```python
from build123d import *

# Parameters (mm, degrees)
EXTRUDE_1_DEPTH          = 66
CUT_EXTRUDE_1_DEPTH      = 66
CUT_EXTRUDE_1_DEPTH_BACK = 66
SKETCH_2_R               = 1.5
SKETCH_4_R               = 3.5
CUT_EXTRUDE_2_DEPTH      = 5
CUT_EXTRUDE_3_DEPTH      = 66
REVOLVE_1_ANGLE          = 110
SKETCH_7_W               = 6.196152423
SKETCH_7_H               = 4
CUT_EXTRUDE_4_DEPTH      = 66


with BuildPart() as part:
    # 草图1 → 凸台-拉伸1 (new body)
    with BuildSketch(Plane(origin=(0, 0, 0), x_dir=(0, 0, -1), z_dir=(1, 0, 0))):
        Polygon((5, 0), (-5, 0), (-25, 34.641016151), (-21.535898385, 36.641016151), (-7.25388745, 11.903847577), (-2, 11.903847577), (-2, 2.803847577), (2, 2.803847577), (2, 11.903847577), (7.25388745, 11.903847577), (21.535898385, 36.641016151), (25, 34.641016151), align=None)
    extrude(amount=EXTRUDE_1_DEPTH)

    # 草图2 → 切除-拉伸1 (cut, two sides: drawn at the far end of the back side and taken through both)
    with BuildSketch(Plane.XY.offset(-CUT_EXTRUDE_1_DEPTH_BACK)):
        with Locations(Location((5, 8.23, 0), (0, 0, 180))):
            Circle(SKETCH_2_R)
        with Locations(Location((50, 8.23, 0), (0, 0, 180))):
            Circle(SKETCH_2_R)
        Polygon((0, 9), (0, 36.641016151), (75.943067727, 36.641016151), (66, 33.022035462), (66, 0), (55.386922379, 29.159191114), align=None)
    extrude(amount=CUT_EXTRUDE_1_DEPTH + CUT_EXTRUDE_1_DEPTH_BACK, mode=Mode.SUBTRACT)

    # 草图4 → 切除-拉伸2 (cut)
    with BuildSketch(Plane(origin=(0, 0, 12), x_dir=(-1, 0, 0), z_dir=(0, 0, -1))):
        with Locations((-5, 8.23)):
            Circle(SKETCH_4_R)
        with Locations(Location((-50, 8.23, 0), (0, 0, 90))):
            Circle(SKETCH_4_R)
    cut_extrude_2 = extrude(amount=CUT_EXTRUDE_2_DEPTH, mode=Mode.SUBTRACT)

    # 镜向1: 切除-拉伸2 across plane
    add(cut_extrude_2.mirror(Plane.XY), mode=Mode.SUBTRACT)

    # 草图5 → 切除-拉伸3 (cut)
    with BuildSketch(Plane(origin=(0, -2.165063509, 3.75), x_dir=(1, 0, 0), z_dir=(0, -0.5000000000000011, 0.8660254037844382))):
        Polygon((32.339646553, 26.483902367), (34.276892815, 21.874447202), (51.364505918, 22.320217945), (58.994441321, 24.725230573), (55.386922379, 36.170133678), align=None)
    cut_extrude_3 = extrude(amount=-CUT_EXTRUDE_3_DEPTH, mode=Mode.SUBTRACT)

    # 镜向2: 切除-拉伸3 across plane
    add(cut_extrude_3.mirror(Plane.XY), mode=Mode.SUBTRACT)

    # 草图6 → 旋转1 (revolve)
    with BuildSketch(Plane.ZY):
        Polygon((-10.196152423, 9), (-2, 9), (-2, 2.803847577), (2, 2.803847577), (2, 9), (10.196152423, 9), (5, 0), (-5, 0), align=None)
    revolve(axis=Axis((0, 9, -10.196152423), (0, 0, -1)), revolution_arc=REVOLVE_1_ANGLE)

    # 草图7 → 切除-拉伸4 (cut)
    with BuildSketch(Plane(origin=(2.892544244, 7.947199994, 0), x_dir=(0.939692620785907, -0.34202014332567265, 0), z_dir=(0.34202014332567265, 0.939692620785907, 0))):
        with Locations((-6.176257502, 0)):
            Rectangle(SKETCH_7_W, SKETCH_7_H)
    extrude(amount=-CUT_EXTRUDE_4_DEPTH, mode=Mode.SUBTRACT)


solid = part.part
```
Design review of the part built by this model. Coordinates are the model's own, in mm. A direction names the side the tool comes from. Coordinates: 2 decimals unless noted, no trailing zeros. Order: outer loops, then holes, each group sorted by start corner. A loop starts at its lowest first (then second) coordinate and runs counter-clockwise, first axis right, second up.
1) Clearance check with flat-ended pins moving along their axes: pin 1 (11 mm diameter, centred on x = 50, y = 8.23, fed in from +Z); pin 2 (10 mm diameter, centred on y = 13, z = -10.5, fed in from -X); pin 3 (4 mm diameter, centred on x = 22, z = 4.5, fed in from +Y); pin 4 (6 mm diameter, centred on y = 18, z = 4.5, fed in from -X). State where each tip first meets the part, or that it passes through.
2) Wall thickness on line 1 along X through (y, z) = (8.23, 9.25); line 2 along X through (y, z) = (7.5, 3); line 3 along Z through (x, y) = (58, 10.75): over which ranges is each line inside the solid? List them lowest first.
3) Mouldability with a two-part tool opening along X and no side actions: class faces 6 (the conical face through (-3.7, 6.33, 7.56)), 7 (the flat face through (28, 7, -2)), 8 (the flat face through (55.126, 19.178, 13.795)) as +X half, -X half, draft (parallel to the pull), parting line (faces both ways), or undercut.
4) Take a section at D-D, the plane x = 29. Give the boundary of the cut face in (y, z).
5) Take a section at B-B, the plane z = 0. Give the boundary of the cut face in (x, y) (3 decimals).
6) Take a section at A-A, the plane y = 13.75. Give the boundary of the cut face in (x, z), and give its area (3 significant figures).
7) Take a section at C-C, the plane x = 50. Give the boundary of the cut face in (y, z), and give its area (3 significant figures).
8) For faces 1 (the flat face through (33.51, 19.35, 13.89)), 2 (the flat face through (50, 10, -7)), 3 (the flat face through (15.431, 14.617, 10.572)), 4 (the cylindrical face through (8.46, 7.71, 8.3)), 5 (the flat face through (32, 2.804, 0)), list the 3-axis set-ups (+Z, -Z, +X, -X, +Y, -Y) from which the entire face can be reached by the end or side of a thin tool; tool diameter is ignored.
Returned:
1. pin 1: stops at z = 12.93
1. pin 2: stops at x = -7.35
1. pin 3: stops at y = 11.9
1. pin 4: passes through
2. line 1: x = -1.45 to 1.5, 8.5 to 46.5, 53.5 to 63
2. line 2: x = -8.87 to 3.69, 6.31 to 48.69, 51.31 to 63.27
2. line 3: z = -11.21 to -2, 2 to 11.21
3. face 6: -X half
3. face 7: draft
3. face 8: undercut
4. outline: (0, -5) - (19.56, -16.29) - (19.56, -11.67) - (11.9, -7.25) - (11.9, -2) - (2.8, -2) - (2.8, 2) - (11.9, 2) - (11.9, 7.25) - (19.56, 11.67) - (19.56, 16.29) - (0, 5) - close
5. outline: (-8.457, 12.078) arc R9 ccw to (-8.055, 4.985) - (-5.822, 11.119) - close; (-3.078, 0.543) arc R9 ccw to (0, 0) - (66, 0) - (64.979, 2.804) - (0, 2.804) arc R6.196 cw to (-2.119, 3.178) - close
6. outline: (13.05, -12.94) - (61, -12.94) - (61, -8.32) - (13.05, -8.32) - close; (13.05, 8.32) - (61, 8.32) - (61, 12.94) - (13.05, 12.94) - close
6. area: 443 mm2
7. outline: (0, -5) - (4.73, -7.73) - (4.73, -7) - (6.73, -7) - (6.73, -2) - (2.8, -2) - (2.8, 2) - (6.73, 2) - (6.73, 7) - (4.73, 7) - (4.73, 7.73) - (0, 5) - close; (9.73, -7) - (11.73, -7) - (11.73, -11.77) - (17.13, -14.89) - (19.13, -11.43) - (11.9, -7.25) - (11.9, -2) - (9.73, -2) - close; (9.73, 2) - (11.9, 2) - (11.9, 7.25) - (19.13, 11.43) - (17.13, 14.89) - (11.73, 11.77) - (11.73, 7) - (9.73, 7) - close
7. area: 153 mm2
8. face 1: +Z, +Y
8. face 2: -Z
8. face 3: +Z, -Z, +Y
8. face 4: +Z
8. face 5: +X, +Y
